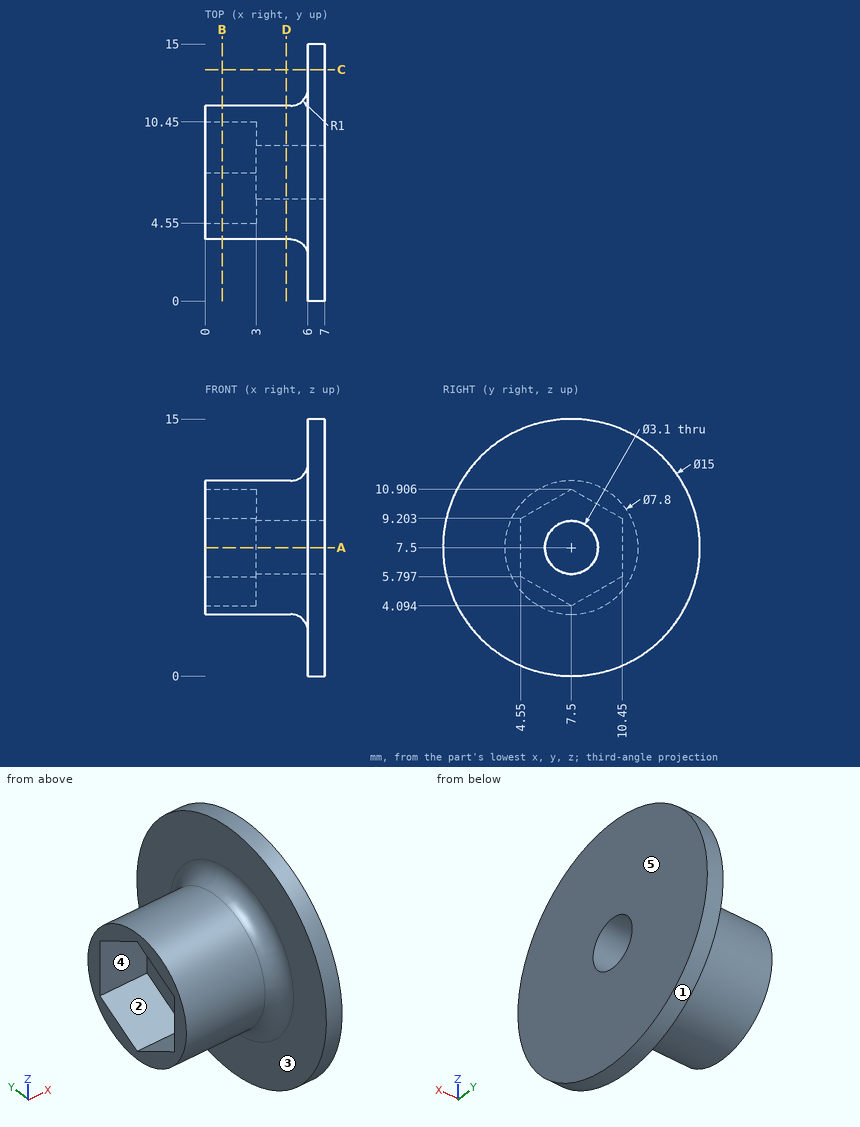
Job drawing, mm, ordinate dimensions from the low corner. One solid piece. A direction names the side the tool comes from. Give positions to 0.01 mm unless a question says otherwise; leave off trailing zeros. Write each loop counter-clockwise with the first axis right and the second up, starting at its lowest first coordinate (ties: lowest second). Pieces come first, ordered by that corner, then holes. Notation, with made-up numbers: M 79,8.25 L 91,8.25 A24 ccw 91,23.25 Z; hole C -9.5,20.25 d3. An arc over 180 degrees is marked long. Put each result on its own line as item: value. Start each with the question number.
(1) Mould opens along Z. For the marked faces 1, 2 and 3 say: +Z half, -Z half, draft (parallel to the pull), parting line (faces both ways), or undercut.
(2) Band-saw the part on A-A, the plane z = 7.5. Write the cut outline in (x, y).
(3) Which spindle directions (+Z, -Z, +X, -X, +Y, -Y) get a long thin tool onto all of the face, cutting with end or side? Do the marked faces 4 and 5. Say none if no direction does.
(4) Band-saw the part on B-B, the plane x = 1. Write the cut outline in (y, z).
(5) Flat gauge pins, fed straight in: pin 1 Ø3.5 at (x, z) = (1, 8.5) entering from -Y; pin 2 Ø2.5 at (x, z) = (2, 8) entering from +Y; pin 3 Ø3 at (x, y) = (2, 9.5) entering from +Z. Where does each tip first touch, or does it go through?
(6) Band-saw the part on D-D, the plane x = 4.75. Write the cut outline in (y, z).
(7) Probe L1, parallel to Y at x = 6.05, z = 7.5; L2, parallel to X at y = 7.25, z = 2; L3, parallel to Y at x = 5, z = 7.5. List the from-to ranges inside material, lowest first.
(8) Band-saw the part on C-C, the plane y = 13.5. Write the cut outline in (x, z).
Response values:
1. face 1: parting line
1. face 2: undercut
1. face 3: draft
2. outline: M 0,3.6 L 5,3.6 A1 cw 6,2.6 L 6,0 L 7,0 L 7,5.95 L 3,5.95 L 3,4.55 L 0,4.55 Z; M 0,10.45 L 3,10.45 L 3,9.05 L 7,9.05 L 7,15 L 6,15 L 6,12.4 A1 cw 5,11.4 L 0,11.4 Z
3. face 4: -X
3. face 5: +Z, -Z, +X, +Y, -Y
4. outline: C 7.5,7.5 d7.8; hole M 4.55,5.8 L 7.5,4.09 L 10.45,5.8 L 10.45,9.2 L 7.5,10.91 L 4.55,9.2 Z
5. pin 1: stops at y = 3.6
5. pin 2: stops at y = 11.4
5. pin 3: stops at z = 11.37
6. outline: C 7.5,7.5 d7.8; hole C 7.5,7.5 d3.1
7. L1: y = 0 to 5.95, 9.05 to 15
7. L2: x = 6 to 7
7. L3: y = 3.6 to 5.95, 9.05 to 11.4
8. outline: M 6,3 L 7,3 L 7,12 L 6,12 Z
